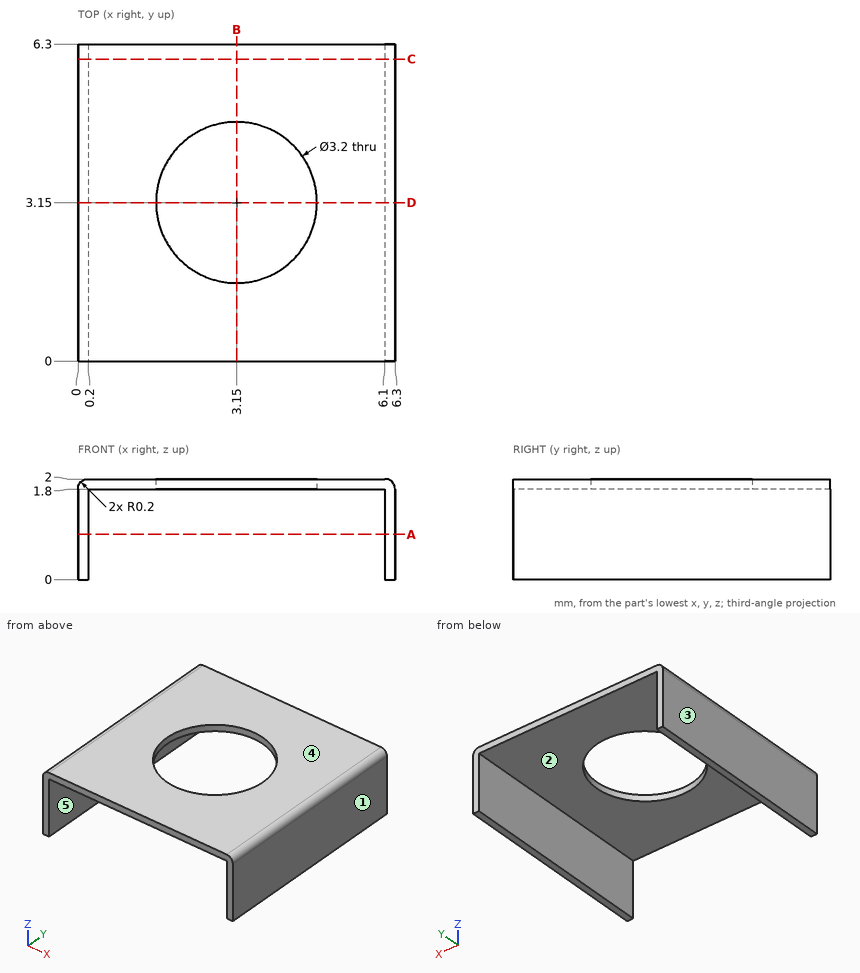
Geometry: see drawing. Coordinates: mm, zero at the bounding-box minimum. A direction names the side the tool comes from. Give positions to 0.01 mm unless a question says otherwise; leave off trailing zeros. Loops run counter-clockwise (first coordinate to the right, second up) from the corner with the lowest first, then second, coordinate; pieces in that order, holes last. Notation, with made-up numbers: (12.5, 9) - (26.5, 9) arc R30 ccw to (26.5, 32) - close; hole circle Ø10 at (86.5, 40.25). An arc over 180 degrees is marked (long way). Use CSV: the item, a comma, the result in double quotes. Start each with the question number.
1. Section A-A (z = 0.9). Output: boundary loops of the cut face in (x, y).
2. Pin query (flat end, axial travel): pin 1 (3 mm diameter, centred on x = 3.15, y = 3.15, fed in from +Z); pin 2 (1 mm diameter, centred on x = 1, y = 1.5, fed in from -Z). Return the tip coordinate at first contact, or that it passes through.
3. Section B-B (x = 3.15). Output: boundary loops of the cut face in (y, z), then the cut area to 3 significant figures.
4. Ray query, L1, parallel to X at y = 5.75, z = 0.85; L2, parallel to Y at x = 3.15, z = 1.9; L3, parallel to Z at x = 4.75, y = 4. Return the intervals inside material, ascending.
5. Reachability of the marked faces 4 and 5 from +Z, -Z, +X, -X, +Y, -Y: full face, straight path, thin tool, end or side. Return the list, or none.
6. Section D-D (y = 3.15). Output: boundary loops of the cut face in (x, z).
7. Draft query along X for the marked faces 1, 2 and 3. Return one class per face: +X half, -X half, draft (parallel to the pull), parting line (faces both ways), or undercut.
8. Section C-C (y = 6). Output: boundary loops of the cut face in (x, z).
Response:
1,outline,"(0, 0) - (0.2, 0) - (0.2, 6.3) - (0, 6.3) - close; (6.1, 0) - (6.3, 0) - (6.3, 6.3) - (6.1, 6.3) - close"
2,pin 1,"through"
2,pin 2,"z = 1.8"
3,outline,"(0, 1.8) - (1.55, 1.8) - (1.55, 2) - (0, 2) - close; (4.75, 1.8) - (6.3, 1.8) - (6.3, 2) - (4.75, 2) - close"
3,area,"0.620 mm²"
4,L1,"0 to 0.2, 6.1 to 6.3"
4,L2,"0 to 1.55, 4.75 to 6.3"
4,L3,"1.8 to 2"
5,face 4,"+Z, +X, -X, +Y, -Y"
5,face 5,"-Z, +Y, -Y"
6,outline,"(0, 0) - (0.2, 0) - (0.2, 1.8) - (1.55, 1.8) - (1.55, 2) - (0.2, 2) arc R0.2 ccw to (0, 1.8) - close; (4.75, 1.8) - (6.1, 1.8) - (6.1, 0) - (6.3, 0) - (6.3, 1.8) arc R0.2 ccw to (6.1, 2) - (4.75, 2) - close"
7,face 1,"+X half"
7,face 2,"undercut"
7,face 3,"-X half"
8,outline,"(0, 0) - (0.2, 0) - (0.2, 1.8) - (6.1, 1.8) - (6.1, 0) - (6.3, 0) - (6.3, 1.8) arc R0.2 ccw to (6.1, 2) - (0.2, 2) arc R0.2 ccw to (0, 1.8) - close"
